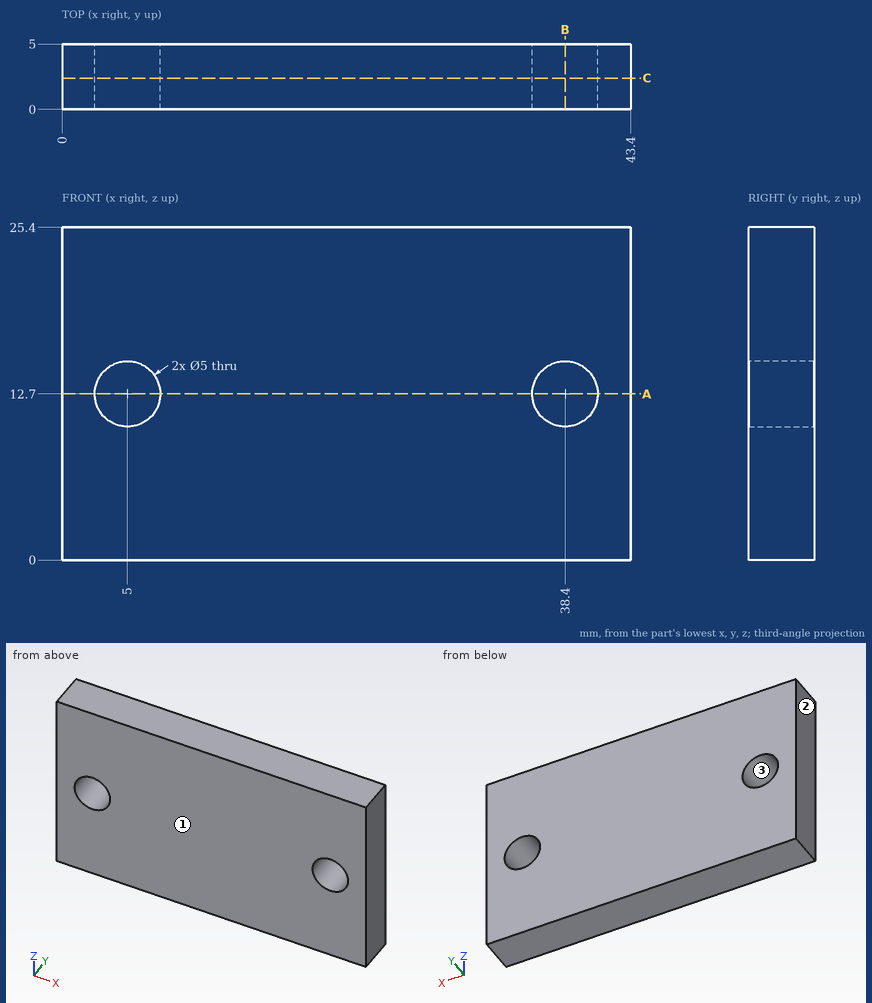
Study the drawing (mm; zero at the part's minimum x, y, z) and answer. Coordinates: 2 decimals unless noted, no trailing zeros. Write each loop counter-clockwise with the first axis right and the second up, starting at its lowest first coordinate (ties: lowest second). Pieces come first, ordered by that corner, then holes.
Q1. A cutting plane is placed at C-C, the plane y = 2.4. Give the vertices of the cut face in (x, z), then the cut area to 3 significant figures.
Q2. Find the intervals of material crossed by line 1 (X direction, y = 3.5, z = 12.7); line 2 (X direction, y = 0.5, z = 11.25), in increasing order.
Q3. A cutting plane is placed at B-B, the plane x = 38.4. Give the vertices of the cut face in (y, z), then the cut area to 3 significant figures.
Q4. Determine the mould class of the marked faces 1, 2 and 3 for opening direction X: released by +X, released by -X, zero draft, split by the parting line, or undercut.
Q5. A cutting plane is placed at A-A, the plane z = 12.7. Give the vertices of the cut face in (x, y), then the cut area to 3 significant figures.
Findings below:
1. outline: (0, 0) - (43.4, 0) - (43.4, 25.4) - (0, 25.4) - close; hole circle Ø5 at (5, 12.7); hole circle Ø5 at (38.4, 12.7)
1. area: 1,060 mm2
2. line 1: x = 0 to 2.5, 7.5 to 35.9, 40.9 to 43.4
2. line 2: x = 0 to 2.96, 7.04 to 36.36, 40.44 to 43.4
3. outline: (0, 0) - (5, 0) - (5, 10.2) - (0, 10.2) - close; (0, 15.2) - (5, 15.2) - (5, 25.4) - (0, 25.4) - close
3. area: 102 mm2
4. face 1: zero draft
4. face 2: released by -X
4. face 3: undercut
5. outline: (0, 0) - (2.5, 0) - (2.5, 5) - (0, 5) - close; (7.5, 0) - (35.9, 0) - (35.9, 5) - (7.5, 5) - close; (40.9, 0) - (43.4, 0) - (43.4, 5) - (40.9, 5) - close
5. area: 167 mm2
